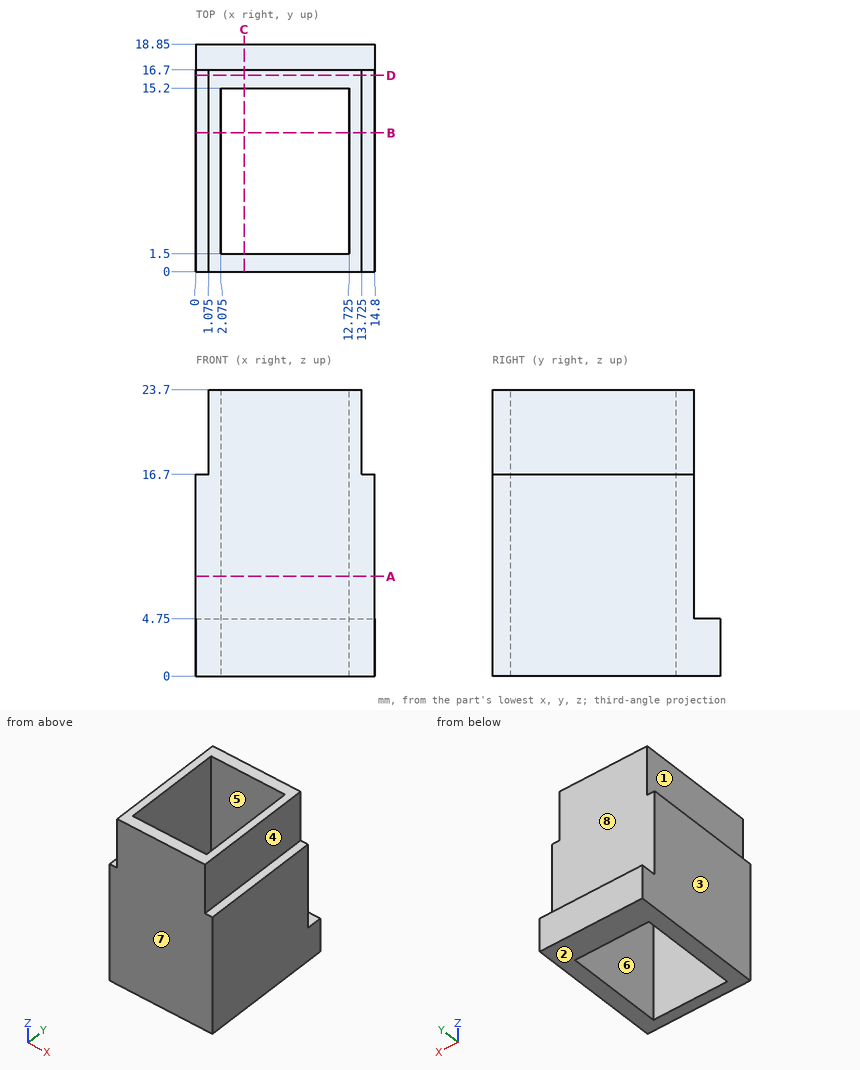
Geometry check sheet. Reference: drawing and pictorial views, mm from the part's lowest x, y, z. A direction names the side the tool comes from. Give positions to 0.01 mm unless a question says otherwise; leave off trailing zeros. Order: outer loops, then holes, each group sorted by start corner. A loop starts at its lowest first (then second) coordinate and runs counter-clockwise, first axis right, second up. Notation, with made-up numbers: (29.5, 85) - (38.5, 85) arc R16 cw to (38.5, 112) - close; hole circle Ø4 at (33.5, -15.5). An arc over 180 degrees is marked (long way). Use one line per item in the form item = value.
1) Sectioned sample at D-D (y = 16.25). Record the boundary of the cut face in (x, z) (3 decimals).
Working result:
outline = (0, 0) - (14.8, 0) - (14.8, 16.7) - (13.725, 16.7) - (13.725, 23.7) - (1.075, 23.7) - (1.075, 16.7) - (0, 16.7) - close
2) Material ranges on probe 1 along X at (y, z) = (5.75, 12.25) (3 decimals); probe 2 along Y at (x, z) = (7, 10.5); probe 3 along X at (y, z) = (9, 17) (3 decimals), recorded low to high. Write a range as from..to.
Working result:
probe_1 = 0..2.075, 12.725..14.8
probe_2 = 0..1.5, 15.2..16.7
probe_3 = 1.075..2.075, 12.725..13.725
3) Draft check along Y on the marked faces 6, 7 and 8. Enter one of: released by +Y, released by -Y, zero draft, split by the parting line, or undercut.
Working result:
face_6 = undercut
face_7 = released by -Y
face_8 = released by +Y
4) Depth check by flat-ended pin: pin 1 Ø2 at (y, z) = (10, 20.5) entering from -X (3 decimals); pin 2 Ø7.5 at (x, z) = (4.5, 13) entering from +Y; pin 3 Ø3.5 at (y, z) = (7.5, 21) entering from +X (3 decimals). Enter the tip coordinate at first touch or a pass-through.
Working result:
pin_1 = 1.075
pin_2 = 16.7
pin_3 = 13.725
5) Access from +Z, -Z, +X, -X, +Y, -Y to the whole of each face (thin tool, end or side, straight path). Record for the marked faces 1, 2, 3, 4 and 5.
Working result:
face_1 = +Z, -X, +Y, -Y
face_2 = -Z, +X, -X, +Y, -Y
face_3 = +Z, -Z, -X, +Y, -Y
face_4 = +Z, +X, +Y, -Y
face_5 = +Z, -Z
6) Sectioned sample at C-C (x = 4). Record the boundary of the cut face in (y, z), and give its area (3 significant figures).
Working result:
outline = (0, 0) - (1.5, 0) - (1.5, 23.7) - (0, 23.7) - close; (15.2, 0) - (18.85, 0) - (18.85, 4.75) - (16.7, 4.75) - (16.7, 23.7) - (15.2, 23.7) - close
area = 81.3 mm^2
7) Sectioned sample at A-A (z = 8.25). Record the boundary of the cut face in (x, y) (3 decimals).
Working result:
outline = (0, 0) - (14.8, 0) - (14.8, 16.7) - (0, 16.7) - close; hole (2.075, 1.5) - (12.725, 1.5) - (12.725, 15.2) - (2.075, 15.2) - close
8) Sectioned sample at B-B (y = 11.5). Record the boundary of the cut face in (x, z) (3 decimals), and give its area (3 significant figures).
Working result:
outline = (0, 0) - (2.075, 0) - (2.075, 23.7) - (1.075, 23.7) - (1.075, 16.7) - (0, 16.7) - close; (12.725, 0) - (14.8, 0) - (14.8, 16.7) - (13.725, 16.7) - (13.725, 23.7) - (12.725, 23.7) - close
area = 83.3 mm^2
